```python
from build123d import *

# Parameters (mm, degrees)
SKETCH2_W           = 193.64
SKETCH2_H           = 180
BOSS_EXTRUDE1_DEPTH = 3.18
CUT_EXTRUDE1_DEPTH  = 133.227927459
SKETCH4_W           = 3.18
SKETCH4_H           = 10
BOSS_EXTRUDE2_DEPTH = 3.18
SKETCH6_R           = 1.47
CUT_EXTRUDE2_DEPTH  = 135.573817662


with BuildPart() as part:
    # Sketch2 → Boss-Extrude1 (new body)
    with BuildSketch(Plane.XY):
        Rectangle(SKETCH2_W, SKETCH2_H)
    extrude(amount=BOSS_EXTRUDE1_DEPTH)

    # Sketch3 → Cut-Extrude1 (cut, through all)
    with BuildSketch(Plane.XY.offset(3.18)):
        Polygon((-5, 90), (5, 90), (5, 86.82), (1.47, 86.82), (1.47, 84.74), (3.25, 84.74), (3.25, 82.14), (1.47, 82.14), (1.47, 80.07), (-1.47, 80.07), (-1.47, 82.14), (-3.25, 82.14), (-3.25, 84.74), (-1.47, 84.74), (-1.47, 86.82), (-5, 86.82), align=None)
        Polygon((1.47, -86.82), (5, -86.82), (5, -90), (-5, -90), (-5, -86.82), (-1.47, -86.82), (-1.47, -84.74), (-3.25, -84.74), (-3.25, -82.14), (-1.47, -82.14), (-1.47, -80.07), (1.47, -80.07), (1.47, -82.14), (3.25, -82.14), (3.25, -84.74), (1.47, -84.74), align=None)
    extrude(amount=-CUT_EXTRUDE1_DEPTH, mode=Mode.SUBTRACT)

    # Sketch4 → Boss-Extrude2 (add)
    with BuildSketch(Plane.ZY.offset(96.82)):
        with Locations((1.59, 0)):
            Rectangle(SKETCH4_W, SKETCH4_H)
    boss_extrude2 = extrude(amount=BOSS_EXTRUDE2_DEPTH)

    # Sketch6 → Cut-Extrude2 (cut, through all)
    with BuildSketch(Plane.XY.offset(3.18)):
        with Locations((-98.25, 0)):
            Circle(SKETCH6_R)
    cut_extrude2 = extrude(amount=-CUT_EXTRUDE2_DEPTH, mode=Mode.SUBTRACT)

    # Mirror1: Boss-Extrude2 across plane
    add(boss_extrude2.mirror(Plane(origin=(0, 0, 0), x_dir=(0, 0, 1), z_dir=(1, 0, 0))))

    # Mirror2: Cut-Extrude2 across plane
    add(cut_extrude2.mirror(Plane(origin=(0, 0, 0), x_dir=(0, 0, 1), z_dir=(1, 0, 0))), mode=Mode.SUBTRACT)


solid = part.part
```
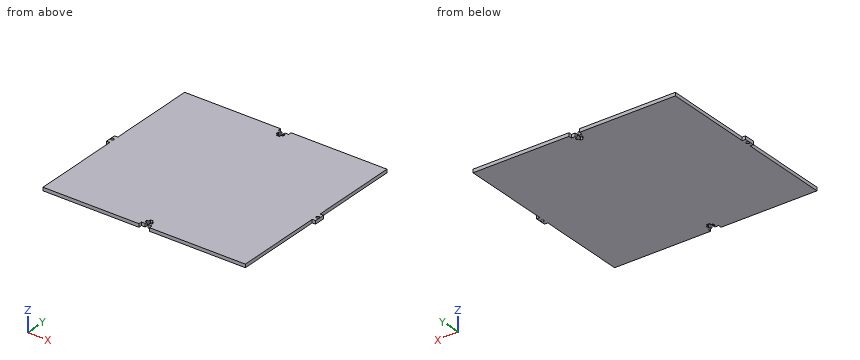
Geometry check sheet. Reference: the model listing, model coordinates, mm. Coordinates: 2 decimals unless noted, no trailing zeros. Order: outer loops, then holes, each group sorted by start corner. A loop starts at its lowest first (then second) coordinate and runs counter-clockwise, first axis right, second up.
Item 1: Section check B-B (y = 10). Enter the section's corners in (x, z).
Item 2: Scan lines: line 1 along Y through (x, z) = (-98.25, 1); line 2 along X through (y, z) = (82, 1.6); line 3 along X through (y, z) = (-71, 0.6). Record each from-to range of solid material in increasing order.
Item 3: Section check A-A (z = 2). Count the separate pieces of the cut face and the enclosed holes in it, plus the area to 3 significant figures.
Item 4: Depth check by flat-ended pin: pin 1 (1.7 mm diameter, centred on y = -86, z = 1, fed in from +X); pin 2 (1.4 mm diameter, centred on x = 2.5, z = 2, fed in from -Y); pin 3 (0.6 mm diameter, centred on y = -86, z = 1, fed in from -X). Enter the tip coordinate at first touch or a pass-through.
Check sheet entries:
1. outline: (-96.82, 0) - (96.82, 0) - (96.82, 3.18) - (-96.82, 3.18) - close
2. line 1: y = -5 to -1.47, 1.47 to 5
2. line 2: x = -96.82 to -1.47, 1.47 to 96.82
2. line 3: x = -96.82 to 96.82
3. separate pieces: 1
3. enclosed holes: 2
3. area: 34,800 mm2
4. pin 1: stops at x = 96.82
4. pin 2: stops at y = -86.82
4. pin 3: stops at x = -96.82
